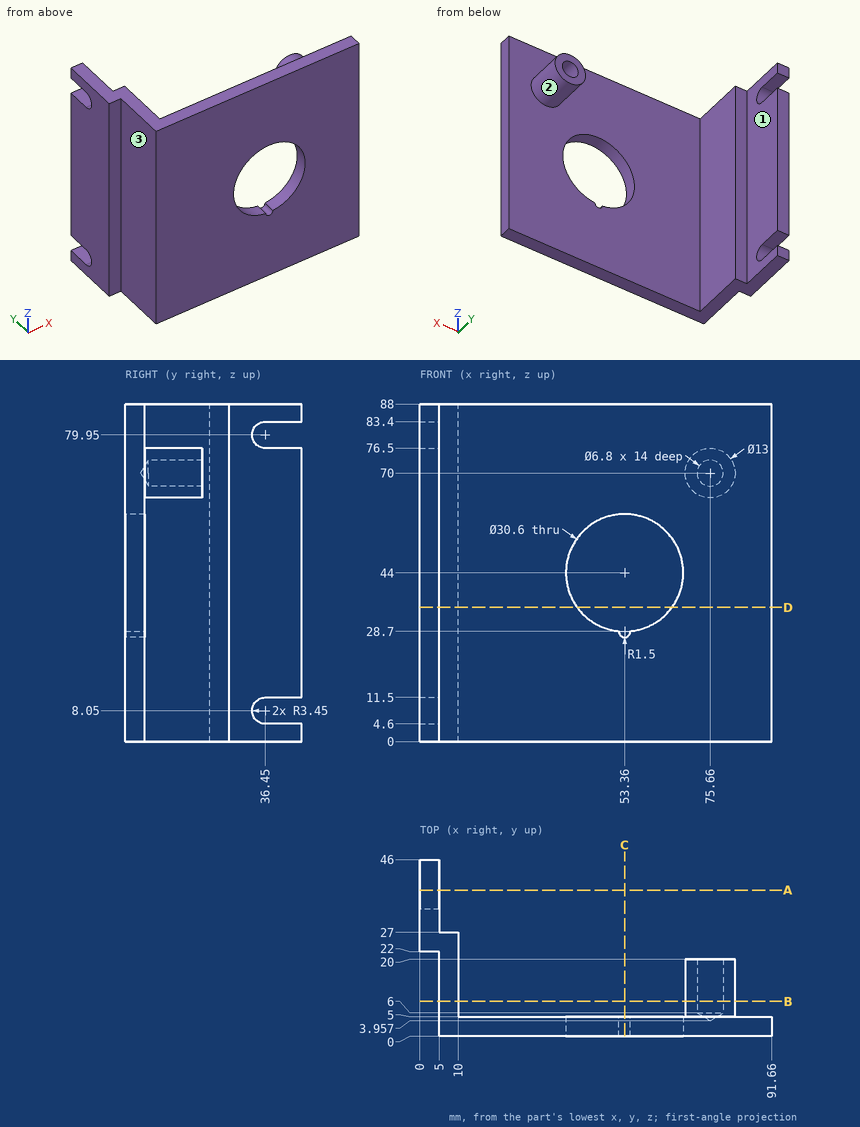
Job drawing, mm, ordinate dimensions from the low corner. One solid piece. Give positions to 0.01 mm unless a question says otherwise; leave off trailing zeros. Loops run counter-clockwise (first coordinate to the right, second up) from the corner with the lowest first, then second, coordinate; pieces in that order, holes last.
Item 1: Drill centre lines: line 1 (X direction, y = 16.75, z = 70); line 2 (Z direction, x = 53.36, y = 3); line 3 (X direction, y = 2, z = 44). Where is each one in solid material? Low to high.
Answers follow:
line 1: x = 5 to 10, 69.16 to 72.26, 79.06 to 82.16
line 2: z = 0 to 27.2, 59.3 to 88
line 3: x = 5 to 38.06, 68.66 to 91.66
Item 2: Slice it at A-A, the plane y = 38. List the corners of the cut face in (x, z), and give its area (3 significant figures).
Answers follow:
outline: (0, 0) - (5, 0) - (5, 4.6) - (0, 4.6) - close; (0, 11.5) - (5, 11.5) - (5, 76.5) - (0, 76.5) - close; (0, 83.4) - (5, 83.4) - (5, 88) - (0, 88) - close
area: 371 mm2
Item 3: Flat gauge pins, fed straight in: pin 1 (24 mm diameter, centred on y = 13, z = 63.5, fed in from -X); pin 2 (10 mm diameter, centred on y = 11, z = 70.5, fed in from -X); pin 3 (11 mm diameter, centred on y = 17.5, z = 47.5, fed in from +X); pin 4 (8 mm diameter, centred on x = 73, y = 21.5, fed in from -Z). Where does each tip first touch, or does it go through?
Answers follow:
pin 1: stops at x = 0
pin 2: stops at x = 5
pin 3: stops at x = 10
pin 4: stops at z = 63.5
Item 4: Slice it at B-B, the plane y = 9. List the corners of the cut face in (x, z), and give its area (3 significant figures).
Answers follow:
outline: (5, 0) - (10, 0) - (10, 88) - (5, 88) - close; circle Ø13 at (75.66, 70); hole circle Ø6.8 at (75.66, 70)
area: 536 mm2
Item 5: Slice it at C-C, the plane x = 53.36. List the corners of the cut face in (y, z).
Answers follow:
outline: (0, 0) - (5, 0) - (5, 27.2) - (0, 27.2) - close; (0, 59.3) - (5, 59.3) - (5, 88) - (0, 88) - close
Item 6: Pull direction X, two halves, no side cores. Call the marked faces 1, 2 and 3: released by +X, released by -X, zero draft, split by the parting line, or undercut.
Answers follow:
face 1: released by +X
face 2: undercut
face 3: released by -X
Item 7: Slice it at D-D, the plane z = 35. List the corners of the cut face in (x, y), and give its area (3 significant figures).
Answers follow:
outline: (0, 22) - (5, 22) - (5, 0) - (40.99, 0) - (40.99, 5) - (10, 5) - (10, 27) - (5, 27) - (5, 46) - (0, 46) - close; (65.73, 0) - (91.66, 0) - (91.66, 5) - (65.73, 5) - close
area: 540 mm2
